Could you check a few things on this model? Use its own coordinates, in mm. A direction names the side the tool comes from. Coordinates: 2 decimals unless noted, no trailing zeros. Loops run counter-clockwise (first coordinate to the right, second up) from the corner with the lowest first, then second, coordinate; pieces in that order, holes last.
1) Imagine slicing it at A-A on z = -12.5. Please give me the cut outline in (x, y).
2) Imagine slicing it at B-B on z = -37. Please give me the cut outline in (x, y), plus the area to 3 significant figures.
3) If I drill on line 1 along Y through (x, z) = (-43.7, -52.5); line 2 along X through (y, z) = (38.5, -50.5); line 3 along Y through (x, z) = (-52, -38), over which ranges is the centre line in solid material (lowest first)?
4) Will these pins go through, and if not, where does the flat tip stop? P1, Ø12, axis at x = -64.5, z = -12, coming from the +Y side; P2, Ø7, axis at y = 114.42, z = -52.5, coming from the -X side.
5) Thinking about a two-plate mould opening in Z: for faces 1 (the face through (-42.4, 69, -32)), 2 (the face through (-46, 63, 0)), 3 (the face through (-44.815, 111.733, -53.096)), which applies, released by +Z, released by -Z, zero draft, split by the parting line, or undercut?
6) Imagine slicing it at C-C on y = 82. Please give me the cut outline in (x, z), plus the area to 3 significant figures.
7) For faces 4 (the face through (-47.162, 73, -32)), 5 (the face through (-77.4, 21, -32)), which set-ups out of +Z, -Z, +X, -X, +Y, -Y let a thin tool reach every point of the face, with its end or its side?
```python
from build123d import *

# Parameters (mm, degrees)
BOSS_EXTRUDE1_DEPTH = 65
SKETCH2_R           = 2.75
CUT_EXTRUDE1_DEPTH  = 10


with BuildPart() as part:
    # Sketch1 → Boss-Extrude1 (new body)
    with BuildSketch(Plane.XY):
        Polygon((-77.4, 19.05), (-42.4, 19.05), (-42.4, 120.65), (-47.1625, 120.65), (-47.1625, 23.8125), (-77.4, 23.8125), align=None)
    extrude(amount=-BOSS_EXTRUDE1_DEPTH)

    # Sketch2 → Cut-Extrude1 (cut)
    with BuildSketch(Plane.ZY.offset(47.1625)):
        with Locations((-12.5, 114.417723435)):
            Circle(SKETCH2_R)
        with Locations((-52.5, 114.417723435)):
            Circle(SKETCH2_R)
    extrude(amount=-CUT_EXTRUDE1_DEPTH, mode=Mode.SUBTRACT)


solid = part.part
```
Filled in:
1. outline: (-77.4, 19.05) - (-42.4, 19.05) - (-42.4, 111.67) - (-47.16, 111.67) - (-47.16, 23.81) - (-77.4, 23.81) - close; (-47.16, 117.17) - (-42.4, 117.17) - (-42.4, 120.65) - (-47.16, 120.65) - close
2. outline: (-77.4, 19.05) - (-42.4, 19.05) - (-42.4, 120.65) - (-47.16, 120.65) - (-47.16, 23.81) - (-77.4, 23.81) - close
2. area: 628 mm2
3. line 1: y = 19.05 to 111.67, 117.17 to 120.65
3. line 2: x = -47.16 to -42.4
3. line 3: y = 19.05 to 23.81
4. P1: stops at y = 23.81
4. P2: stops at x = -47.16
5. face 1: zero draft
5. face 2: released by +Z
5. face 3: undercut
6. outline: (-47.16, -65) - (-42.4, -65) - (-42.4, 0) - (-47.16, 0) - close
6. area: 310 mm2
7. face 4: +Z, -Z, -X, +Y
7. face 5: +Z, -Z, -X, +Y, -Y
